from build123d import *

# Parameters (mm, degrees)
BASPROSKE_W             = 10
BASPROSKE_H             = 24.75
TOOTHCUT_DEPTH          = 37.402266413
TEETHCUTS_COUNT         = 11
TEETHCUTS_ANGLE         = 180
HUBNEAONESKE_R          = 15
HUBNEARONE_DEPTH        = 7.0000508
BORSKE_R                = 5
BORE_DEPTH              = 10.0000508
KEYSKE_W                = 4
KEYSKE_H                = 6.8
KEYWAY_DEPTH            = 10.0000508
ESQUISSE1_W             = 100
ESQUISSE1_H             = 10
BOSS_EXTRU_1_DEPTH      = 10
ESQUISSE2_R             = 3
ENL_V_MAT_EXTRU_2_DEPTH = 10


with BuildPart() as part:
    # BasProSke → Base-Revolve (revolve)
    with BuildSketch(Plane(origin=(0, 0, 0), x_dir=(1, 0, 0), z_dir=(0, 1, 0)), mode=Mode.PRIVATE) as base_revolve_sk:
        with Locations((5, 12.375)):
            Rectangle(BASPROSKE_W, BASPROSKE_H)
    revolve(base_revolve_sk.sketch.rotate(Axis((-10, 0, 0), (1, 0, 0)), 180), axis=Axis((-10, 0, 0), (1, 0, 0)))

    # TooCutSke → ToothCut (cut, through all)
    with BuildSketch(Plane(origin=(0, 0, 0), x_dir=(0, 0, -1), z_dir=(1, 0, 0))):
        with BuildLine():
            ThreePointArc((1.111948432, 19.655071939), (0, 19.6865), (-1.111948432, 19.655071939))
            ThreePointArc((-1.111948432, 19.655071939), (-1.832349961, 22.271720111), (-3.300041734, 24.55463642))
            ThreePointArc((-3.300041734, 24.55463642), (0, 24.7754), (3.300041734, 24.55463642))
            ThreePointArc((3.300041734, 24.55463642), (1.832349961, 22.271720111), (1.111948432, 19.655071939))
        make_face()
    toothcut = extrude(amount=TOOTHCUT_DEPTH, mode=Mode.SUBTRACT)

    # TeethCuts: ToothCut ×11 about axis
    teethcuts_axis = Axis((-10, 0, 0), (1, 0, 0))
    for i in range(1, TEETHCUTS_COUNT):
        add(toothcut.rotate(teethcuts_axis, i * TEETHCUTS_ANGLE / (TEETHCUTS_COUNT - 1)), mode=Mode.SUBTRACT)

    # HubNeaOneSke → HubNearOne (add)
    with BuildSketch(Plane.ZY):
        with Locations(Location((0, 0, 0), (0, 0, 180))):
            Circle(HUBNEAONESKE_R)
    extrude(amount=HUBNEARONE_DEPTH)

    # BorSke → Bore (cut, symmetric)
    with BuildSketch(Plane(origin=(0, 0, 0), x_dir=(0, 0, -1), z_dir=(1, 0, 0))):
        with Locations(Location((0, 0, 0), (0, 0, 180))):
            Circle(BORSKE_R)
    extrude(amount=BORE_DEPTH, both=True, mode=Mode.SUBTRACT)

    # KeySke → Keyway (cut, symmetric)
    with BuildSketch(Plane(origin=(0, 0, 0), x_dir=(0, 0, -1), z_dir=(1, 0, 0))):
        with Locations((0, 3.4)):
            Rectangle(KEYSKE_W, KEYSKE_H)
    extrude(amount=KEYWAY_DEPTH, both=True, mode=Mode.SUBTRACT)

    # Esquisse1 → Boss.-Extru.1 (add)
    with BuildSketch(Plane(origin=(10, 0, 0), x_dir=(0, 0, -1), z_dir=(1, 0, 0))):
        with Locations((74.239688529, 0)):
            Rectangle(ESQUISSE1_W, ESQUISSE1_H)
    extrude(amount=-BOSS_EXTRU_1_DEPTH)

    # Esquisse2 → Enlèv. mat.-Extru.2 (cut)
    with BuildSketch(Plane.ZY):
        with Locations((-118.101402352, 0)):
            Circle(ESQUISSE2_R)
    extrude(amount=-ENL_V_MAT_EXTRU_2_DEPTH, mode=Mode.SUBTRACT)


solid = part.part
Geometry: final body of the model. Coordinates: model frame, mm. A direction names the side the tool comes from. Round coordinates to 2 decimals unless told otherwise and drop trailing zeros. Loops run counter-clockwise (first coordinate to the right, second up) from the corner with the lowest first, then second, coordinate; pieces in that order, holes last. Notation, with made-up numbers: (25, 54.25) -> (82, 54.25) arc R35 cw to (82, 87.25) -> close; hole circle Ø6 at (-23, -25). An arc over 180 degrees is marked (long way). One line per question, with ' | ' between items. Start each with the question number.
1. Set-up query: faces 5 (the face through (4.93, 14.59, 16.95)), 6 (the face through (4.93, -21.695, 5.145)), 7 (the face through (4.9, 16.9, 14.5)), 8 (the face through (-3.45, -12.65, -8.06)), 9 (the face through (4.93, -20.63, 8.64)). Return all of +Z, -Z, +X, -X, +Y, -Y with unobstructed straight access to the full face (end or side cutting, diameter ignored); none if empty.
2. Contact query for flat-ended pins moving along their axis: pin 1 (6 mm diameter, centred on x = 2.5, z = -35.5, fed in from +Y); pin 2 (5 mm diameter, centred on y = 0, z = -118.1, fed in from -X); pin 3 (4 mm diameter, centred on x = -5, y = 2, fed in from +Z); pin 4 (1 mm diameter, centred on x = 1.5, y = 1.5, fed in from +Z). Output: stop coordinate, or through.
3. Section C-C on x = 1.75. Count the separate pieces of the cut face and the enclosed holes in it, and give its area (3 significant figures).
4. Section A-A on x = -4. Output: boundary loops of the cut face in (y, z), and give its area (3 significant figures).
5. Line query: line 1 along Y through (x, z) = (2, 0); line 2 along Y through (x, z) = (1.5, -76); line 3 along Z through (x, y) = (5.5, 6.5). Output: solid intervals per line, ascending. Write a range as [from, to].
6. Section B-B on z = -74. Output: boundary loops of the cut face in (x, y).
7. Mould query, pull axis Z, two halves, no side actions, for faces 1 (the face through (4.93, 8.64, 20.63)), 2 (the face through (5.07, -18.25, -16.72)), 3 (the face through (5, -5, -74)), 4 (the face through (4.93, 21.77, 5.137)). Classes: pulls with the +Z half, pulls with the -Z half, needs draft (parallel to the pull), parting line crosses it, or undercut.
Returned:
1) face 5: +Z, +X, -X | face 6: +X, -X | face 7: +X, -X, +Y | face 8: -X | face 9: +X, -X, -Y
2) pin 1: stops at y = 5 | pin 2: passes through | pin 3: stops at z = 15 | pin 4: stops at z = 22.63
3) separate pieces: 1 | enclosed holes: 2 | area: 2,590 mm2
4) outline: circle Ø30 at (0, 0); hole (4.58, -2) -> (6.8, -2) -> (6.8, 2) -> (4.58, 2) arc R5 ccw (long way) to start | area: 621 mm2
5) line 1: y = [-19.69, -5], [6.8, 19.69] | line 2: y = [-5, 5] | line 3: z = [-23.88, -2], [2, 18.58]
6) outline: (0, -5) -> (10, -5) -> (10, 5) -> (0, 5) -> close
7) face 1: pulls with the +Z half | face 2: pulls with the -Z half | face 3: needs draft | face 4: undercut
